For this review, take the finished solid that the model builds, in its own axes (mm). Face numbers are marked on the shaded views. Coordinates: 2 decimals unless noted, no trailing zeros. Write each loop counter-clockwise with the first axis right and the second up, starting at its lowest first coordinate (ties: lowest second). Pieces come first, ordered by that corner, then holes. Notation, with made-up numbers: (82.5, -1.75) -> (101.5, -1.75) arc R29 ccw to (101.5, 22.25) -> close; hole circle Ø8 at (-27.5, -10.75). An arc over 180 degrees is marked (long way). Put each result on its own line as item: value. Start each with the question number.
Item 1: Consider section A-A on y = 61.5. Give the boundary of the cut face in (x, z), and give its area (3 significant figures).
Item 2: Insertion check: P1, Ø20, axis at x = 3.5, y = 232, coming from the -Z side; P2, Ø22.5, axis at x = 3, y = 89, coming from the -Z side; P3, Ø12, axis at x = -9.5, z = -20.5, coming from the -Y side; P4, Ø9, axis at x = 0, y = 40, coming from the -Z side. Each pin has a flat end and moves straight along its axis. Give the tip position at first contact, or say it passes through.
Item 3: Consider section C-C on y = 233. Give the boundary of the cut face in (x, z).
Item 4: Consider section B-B on x = -26. Give the boundary of the cut face in (y, z).
Item 5: The part is to be moulded in two halves that separate along X. For the marked faces 1, 2, 3 and 4, say which applies: +X half, -X half, draft (parallel to the pull), parting line (faces both ways), or undercut.
Item 6: Consider section D-D on z = 3.5. Give the boundary of the cut face in (x, y).
Item 7: To check wall thickness, follow L1, parallel to Y at x = 0, z = 9.3; L2, parallel to X at y = 67, z = 2.5; L3, parallel to Z at x = 0.5, y = 151. State the ranges of each line that lie inside material, in increasing order.
```python
from build123d import *

# Parameters (mm, degrees)
SKETCH1_W           = 80
SKETCH1_H           = 20
BOSS_EXTRUDE1_DEPTH = 200
SKETCH2_W           = 75
SKETCH2_H           = 16
CUT_EXTRUDE1_DEPTH  = 190
SKETCH3_R           = 7.5
CUT_EXTRUDE3_DEPTH  = 10
SKETCH4_W           = 80
SKETCH4_H           = 20
SKETCH4_W_2         = 75
SKETCH4_H_2         = 16
BOSS_EXTRUDE2_DEPTH = 50
SKETCH5_R           = 5
CUT_EXTRUDE4_DEPTH  = 10
REVOLVE1_ANGLE      = 180
SKETCH8_R           = 10
CUT_EXTRUDE5_DEPTH  = 10
SKETCH7_R           = 5
BOSS_EXTRUDE3_DEPTH = 15
SKETCH9_R           = 4
CUT_EXTRUDE6_DEPTH  = 30


with BuildPart() as part:
    # Sketch1 → Boss-Extrude1 (new body)
    with BuildSketch(Plane(origin=(0, 0, 0), x_dir=(1, 0, 0), z_dir=(0, 1, 0))):
        Rectangle(SKETCH1_W, SKETCH1_H)
    extrude(amount=BOSS_EXTRUDE1_DEPTH)

    # Sketch2 → Cut-Extrude1 (cut)
    with BuildSketch(Plane(origin=(0, 200, 0), x_dir=(1, 0, 0), z_dir=(0, 1, 0))):
        Rectangle(SKETCH2_W, SKETCH2_H)
    extrude(amount=-CUT_EXTRUDE1_DEPTH, mode=Mode.SUBTRACT)

    # Sketch3 → Cut-Extrude3 (cut)
    with BuildSketch(Plane(origin=(0, 0, -10), x_dir=(-1, 0, 0), z_dir=(0, 0, -1))):
        with Locations(Location((0, 40, 0), (0, 0, 180))):
            Circle(SKETCH3_R)
    extrude(amount=-CUT_EXTRUDE3_DEPTH, mode=Mode.SUBTRACT)

    # Sketch4 → Boss-Extrude2 (add)
    with BuildSketch(Plane(origin=(0, 200, 0), x_dir=(1, 0, 0), z_dir=(0, 1, 0))):
        Rectangle(SKETCH4_W, SKETCH4_H)
        Rectangle(SKETCH4_W_2, SKETCH4_H_2, mode=Mode.SUBTRACT)
    extrude(amount=BOSS_EXTRUDE2_DEPTH)

    # Sketch5 → Cut-Extrude4 (cut)
    with BuildSketch(Plane.XY.offset(10)):
        with Locations((0, 220)):
            Circle(SKETCH5_R)
    extrude(amount=-CUT_EXTRUDE4_DEPTH, mode=Mode.SUBTRACT)

    # Sketch6 → Revolve1 (revolve)
    with BuildSketch(Plane.XY.offset(10)):
        Polygon((0, 250), (40, 250), (40, 200), (0, 200), (0, 205), (35, 205), (35, 245), (0, 245), align=None)
    revolve(axis=Axis((0, 0, 10), (0, 1, 0)), revolution_arc=REVOLVE1_ANGLE)

    # Sketch8 → Cut-Extrude5 (cut)
    with BuildSketch(Plane.XY.offset(10)):
        with Locations((0, 30)):
            Circle(SKETCH8_R)
    extrude(amount=-CUT_EXTRUDE5_DEPTH, mode=Mode.SUBTRACT)

    # Sketch7 → Boss-Extrude3 (add)
    with BuildSketch(Plane.XZ.offset(-200)):
        with Locations(Location((0, -20, 0), (0, 0, 180))):
            Circle(SKETCH7_R)
    extrude(amount=BOSS_EXTRUDE3_DEPTH)

    # Sketch9 → Cut-Extrude6 (cut)
    with BuildSketch(Plane.XZ.offset(-185)):
        with Locations((0, -20)):
            Circle(SKETCH9_R)
    extrude(amount=-CUT_EXTRUDE6_DEPTH, mode=Mode.SUBTRACT)


solid = part.part
```
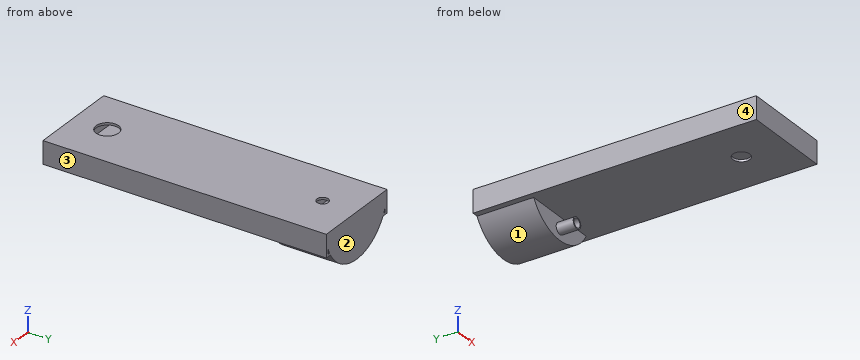
Return value:
1. outline: (-40, -10) -> (40, -10) -> (40, 10) -> (-40, 10) -> close; hole (-37.5, -8) -> (37.5, -8) -> (37.5, 8) -> (-37.5, 8) -> close
1. area: 400 mm^2
2. P1: z = -30
2. P2: z = -10
2. P3: y = 185
2. P4: z = 8
3. outline: (-40, -10) -> (-34.64, -10) arc R40 ccw to (34.64, -10) -> (40, -10) -> (40, 10) -> (-40, 10) -> close; hole (-37.5, -8) -> (-35.72, -8) arc R40 cw to (-37.5, -3.92) -> close; hole (-34.94, 8) arc R35 ccw to (-30.02, -8) -> (30.02, -8) arc R35 ccw to (34.94, 8) -> close; hole (-28.72, -10) arc R35 ccw to (28.72, -10) -> close; hole (35.72, -8) -> (37.5, -8) -> (37.5, -3.92) arc R40 cw to start
4. outline: (0, -10) -> (200, -10) -> (200, -20.4) -> (250, -20.4) -> (250, 10) -> (0, 10) -> close; hole (10, -8) -> (200, -8) -> (200, 8) -> (10, 8) -> close; hole (205, -13.43) -> (245, -13.43) -> (245, -10) -> (205, -10) -> close; hole (205, -8) -> (245, -8) -> (245, 8) -> (205, 8) -> close
5. face 1: parting line
5. face 2: draft
5. face 3: +X half
5. face 4: -X half
6. outline: (-40, 0) -> (40, 0) -> (40, 250) -> (-40, 250) -> close; hole (-37.5, 10) -> (37.5, 10) -> (37.5, 200) -> (-37.5, 200) -> close; hole (-34.39, 205) -> (34.39, 205) -> (34.39, 245) -> (-34.39, 245) -> close
7. L1: 0 to 20, 40 to 215, 225 to 250
7. L2: -40 to -37.5, 37.5 to 40
7. L3: -10 to -8, 8 to 10
